Part model, mm, in its own coordinate system. Face numbers are marked on the shaded views. Coordinates: 2 decimals unless noted, no trailing zeros. Loops run counter-clockwise (first coordinate to the right, second up) from the corner with the lowest first, then second, coordinate; pieces in that order, holes last. Notation, with made-up numbers: M 43,-6 L 92,-6 A30 cw 92,26 Z; hole C 38.25,10 d10. An arc over 180 degrees is marked long. Answer as a JSON object with one key per item and string values. Group by question number.
1. Drill centre lines: L1, parallel to Z at x = 5.25, y = 3.75; L2, parallel to Y at x = -0.75, z = 7.5; L3, parallel to Y at x = 4.5, z = 2. Where is each one in solid material? Low to high.
2. Drop flat-ended pins along their axis: pin 1 Ø1.5 at (x, z) = (5.5, 31.5) entering from -Y; pin 2 Ø12 at (y, z) = (3.5, 30.5) entering from +X; pin 3 Ø6 at (x, y) = (3, -6.5) entering from +Z. Give the stop position or say it passes through.
3. Saw through at A-A on x = 0. Write the cut outline in (y, z).
4. Saw through at B-B on z = 23. Write the cut outline in (x, y).
5. Mould opens along X. For the marked faces 1 and 2 say: released by +X, released by -X, zero draft, split by the parting line, or undercut.
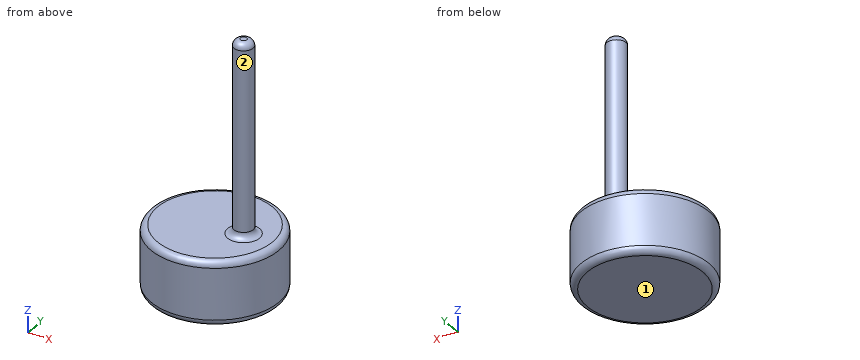
from build123d import *

# Parameters (mm, degrees)
SKETCH1_R           = 10
BOSS_EXTRUDE1_DEPTH = 10
SKETCH2_R           = 1.5
BOSS_EXTRUDE2_DEPTH = 30
FILLET1_R           = 1


with BuildPart() as part:
    # Sketch1 → Boss-Extrude1 (new body)
    with BuildSketch(Plane.XY):
        Circle(SKETCH1_R)
    extrude(amount=BOSS_EXTRUDE1_DEPTH)

    # Sketch2 → Boss-Extrude2 (add)
    with BuildSketch(Plane.XY.offset(10)):
        with Locations((4.5, 0)):
            Circle(SKETCH2_R)
    extrude(amount=BOSS_EXTRUDE2_DEPTH)

    # Fillet1
    fillet1_edges = [part.edges().sort_by_distance(p)[0] for p in [
        (-10, 0, 0),
        (-10, 0, 10),
        (3, 0, 10),
        (3, 0, 40),
    ]]
    fillet(fillet1_edges, radius=FILLET1_R)


solid = part.part
Outcome:
{
 "1": {"L1": "z = 0 to 10", "L2": "y = -9.97 to 9.97", "L3": "y = -8.93 to 8.93"},
 "2": {"pin 1": "stops at y = -1.48", "pin 2": "stops at x = 6", "pin 3": "stops at z = 10"},
 "3": {"outline": "M -10,1 A1 ccw -9,0 L 9,0 A1 ccw 10,1 L 10,9 A1 ccw 9,10 L -9,10 A1 ccw -10,9 Z"},
 "4": {"outline": "C 4.5,0 d3"},
 "5": {"face 1": "zero draft", "face 2": "split by the parting line"}
}
